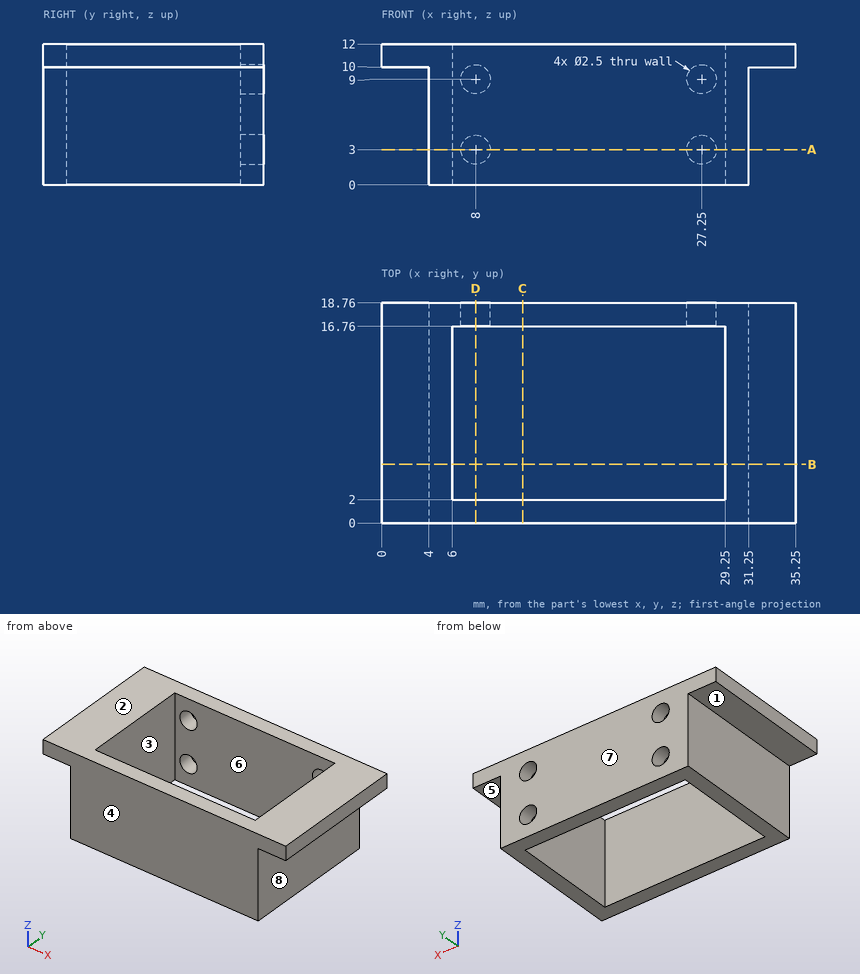
Study the drawing (mm; zero at the part's minimum x, y, z) and answer. A direction names the side the tool comes from. Give positions to 0.01 mm unless a question says otherwise; leave off trailing zeros. Write each loop counter-clockwise with the first axis right and the second up, starting at its lowest first coordinate (ties: lowest second). Pieces come first, ordered by that corner, then holes.
(1) The part is cut by section D-D on x = 8. Write down the section's boundary in (y, z), plus the area to 3 significant figures.
Final values:
outline: (0, 0) - (2, 0) - (2, 12) - (0, 12) - close; (16.76, 0) - (18.76, 0) - (18.76, 1.75) - (16.76, 1.75) - close; (16.76, 4.25) - (18.76, 4.25) - (18.76, 7.75) - (16.76, 7.75) - close; (16.76, 10.25) - (18.76, 10.25) - (18.76, 12) - (16.76, 12) - close
area: 38.0 mm2
(2) The mould has two halves that part along X. Classify the marked faces 6, 7 and 8: pulls with the +X half, pulls with the -X half, needs draft (parallel to the pull), parting line crosses it, or undercut.
Final values:
face 6: undercut
face 7: needs draft
face 8: pulls with the +X half
(3) The part is cut by section C-C on x = 12. Write down the section's boundary in (y, z).
Final values:
outline: (0, 0) - (2, 0) - (2, 12) - (0, 12) - close; (16.76, 0) - (18.76, 0) - (18.76, 12) - (16.76, 12) - close
(4) Flat-ended cylindrical pins translate along their axes: pin 1 Ø2 at (x, y) = (8, 14) entering from +Z; pin 2 Ø5 at (y, z) = (9, 6) entering from -X; pin 3 Ø4.5 at (x, y) = (34, 5) entering from -Z; pin 4 Ø2 at (x, z) = (27.25, 3) entering from +Y. Find the tip coordinate at first contact, or state that the pin passes through.
Final values:
pin 1: passes through
pin 2: stops at x = 4
pin 3: stops at z = 10
pin 4: stops at y = 2
(5) The part is cut by section B-B on y = 5. Write down the section's boundary in (x, z), plus the area to 3 significant figures.
Final values:
outline: (0, 10) - (4, 10) - (4, 0) - (6, 0) - (6, 12) - (0, 12) - close; (29.25, 0) - (31.25, 0) - (31.25, 10) - (35.25, 10) - (35.25, 12) - (29.25, 12) - close
area: 64.0 mm2
(6) Which of the six approach directions +Z, -Z, +X, -X, +Y, -Y give full straight-line access (tool end or side, diameter ignored) to the marked faces 1, 2, 3, 4 and 5?
Final values:
face 1: -Z, -X, +Y, -Y
face 2: +Z, +X, -X, +Y, -Y
face 3: +Z, -Z
face 4: +Z, -Z, +X, -X, -Y
face 5: -Z, +X, +Y, -Y
(7) Straight lines are drawn through the part: line 1 (X direction, y = 17.9, z = 3); line 2 (X direction, y = 11.25, z = 4.75); line 3 (Y direction, x = 22.5, z = 9.25). For each, find the intervals that lie inside material, in ascending order.
Final values:
line 1: x = 4 to 6.75, 9.25 to 26, 28.5 to 31.25
line 2: x = 4 to 6, 29.25 to 31.25
line 3: y = 0 to 2, 16.76 to 18.76
(8) The part is cut by section A-A on z = 3. Write down the section's boundary in (x, y), plus the area to 3 significant figures.
Final values:
outline: (4, 0) - (31.25, 0) - (31.25, 18.76) - (28.5, 18.76) - (28.5, 16.76) - (29.25, 16.76) - (29.25, 2) - (6, 2) - (6, 16.76) - (6.75, 16.76) - (6.75, 18.76) - (4, 18.76) - close; (9.25, 16.76) - (26, 16.76) - (26, 18.76) - (9.25, 18.76) - close
area: 158 mm2
